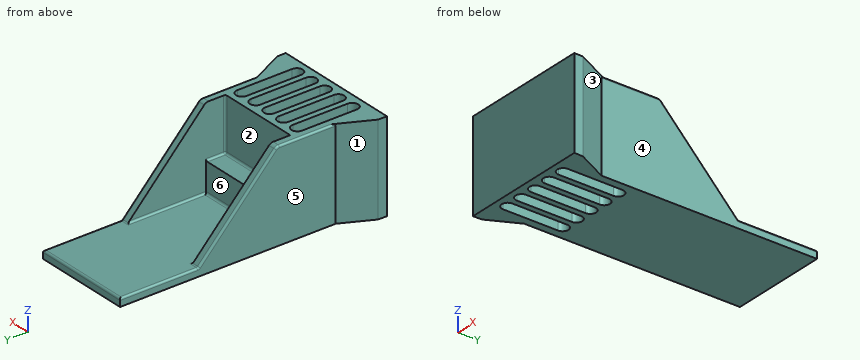
from build123d import *

# Parameters (mm, degrees)
SKETCH_1_W             = 50
SKETCH_1_H             = 46
EXTRUDE_1_DEPTH        = 40
EXTRUDE_2_DEPTH        = 10
SKETCH_8_W             = 42
SKETCH_8_H             = 10
EXTRUDE_5_DEPTH        = 15
SKETCH_3_W             = 50
SKETCH_3_H             = 4
EXTRUDE_3_DEPTH        = 80
SKETCH_4_W             = 70
SKETCH_4_H             = 46
SKETCH_5_W             = 50
SKETCH_5_H             = 46
EXTRUDE_4_DEPTH        = 4
FILLET_2_R             = 3
CHAMFER_1_SIZE2        = 2.113879869
CHAMFER_1_SIZE         = 5
CHAMFER_1_EDGE_2_SIZE2 = 5
CHAMFER_1_EDGE_2_SIZE  = 2.113879869
FILLET_4_R             = 1
CUT_EXTRUDE_1_DEPTH    = 47.0000001
FILLET_5_R             = 1


with BuildPart() as part:
    # 草图1 → 凸台-拉伸1 (new body)
    with BuildSketch(Plane(origin=(0, 0, 0), x_dir=(1, 0, 0), z_dir=(0, 1, 0))):
        with Locations((0, 2)):
            Rectangle(SKETCH_1_W, SKETCH_1_H)
    extrude(amount=EXTRUDE_1_DEPTH)

    # 草图2 → 凸台-拉伸2 (add)
    with BuildSketch(Plane(origin=(0, 40, 0), x_dir=(1, 0, 0), z_dir=(0, 1, 0))):
        Polygon((-25, 25), (-25, -21), (-21, -21), (-21, 21), (21, 21), (21, -21), (25, -21), (25, 25), align=None)
    extrude(amount=EXTRUDE_2_DEPTH)

    # 草图8 → 凸台-拉伸5 (add)
    with BuildSketch(Plane.XY.offset(-21)):
        with Locations((0, 45)):
            Rectangle(SKETCH_8_W, SKETCH_8_H)
    extrude(amount=EXTRUDE_5_DEPTH)

    # 草图3 → 凸台-拉伸3 (add)
    with BuildSketch(Plane(origin=(0, 50, 0), x_dir=(1, 0, 0), z_dir=(0, 1, 0))):
        with Locations((0, 23)):
            Rectangle(SKETCH_3_W, SKETCH_3_H)
    extrude(amount=EXTRUDE_3_DEPTH)

    # 草图4 → 放样2 section 0
    with BuildSketch(Plane.XZ):
        with Locations((0, -2)):
            Rectangle(SKETCH_4_W, SKETCH_4_H)
    # 草图5 → 放样2 section 1
    with BuildSketch(Plane(origin=(0, 20, 0), x_dir=(1, 0, 0), z_dir=(0, 1, 0))):
        with Locations((0, 2)):
            Rectangle(SKETCH_5_W, SKETCH_5_H)
    loft()

    # 草图6 → 凸台-拉伸4 (add)
    with BuildSketch(Plane.ZY.offset(25)):
        Polygon((-21, 90), (21, 50), (-21, 50), align=None)
    extrude_4 = extrude(amount=-EXTRUDE_4_DEPTH)

    # 镜向2: 凸台-拉伸4 across plane
    add(extrude_4.mirror(Plane(origin=(0, 0, 0), x_dir=(0, 0, 1), z_dir=(1, 0, 0))))

    # 圆角2
    fillet_2_edges = [part.edges().sort_by_distance(p)[0] for p in [
        (23, 50, 21),
        (-23, 50, 21),
    ]]
    fillet(fillet_2_edges, radius=FILLET_2_R)

    # 倒角1
    chamfer_1_edges = [part.edges().sort_by_distance(p)[0] for p in [
        (35, 0, -2),
    ]]
    chamfer(chamfer_1_edges, length=CHAMFER_1_SIZE, length2=CHAMFER_1_SIZE2)

    # 倒角1 edge 2
    chamfer_1_edge_2_edges = [part.edges().sort_by_distance(p)[0] for p in [
        (-35, 0, -2),
    ]]
    chamfer(chamfer_1_edge_2_edges, length=CHAMFER_1_EDGE_2_SIZE, length2=CHAMFER_1_EDGE_2_SIZE2)

    # 圆角4
    fillet_4_edges = [part.edges().sort_by_distance(p)[0] for p in [
        (21, 40, 7.5),
    ]]
    fillet(fillet_4_edges, radius=FILLET_4_R)

    # 草图7 → 切除-拉伸1 (cut, through all)
    with BuildSketch(Plane.XY.offset(21)):
        with BuildLine():
            Line((-21, 34), (-21, 6))
            ThreePointArc((-21, 6), (-18, 3), (-15, 6))
            Line((-15, 6), (-15, 34))
            ThreePointArc((-15, 34), (-18, 37), (-21, 34))
        make_face()
        with BuildLine():
            Line((-12, 34), (-12, 6))
            ThreePointArc((-12, 6), (-9, 3), (-6, 6))
            Line((-6, 6), (-6, 34))
            ThreePointArc((-6, 34), (-9, 37), (-12, 34))
        make_face()
        with BuildLine():
            Line((-3, 34), (-3, 6))
            ThreePointArc((-3, 6), (0, 3), (3, 6))
            Line((3, 6), (3, 34))
            ThreePointArc((3, 34), (0, 37), (-3, 34))
        make_face()
        with BuildLine():
            Line((6, 34), (6, 6))
            ThreePointArc((6, 6), (9, 3), (12, 6))
            Line((12, 6), (12, 34))
            ThreePointArc((12, 34), (9, 37), (6, 34))
        make_face()
        with BuildLine():
            Line((15, 34), (15, 6))
            ThreePointArc((15, 6), (18, 3), (21, 6))
            Line((21, 6), (21, 34))
            ThreePointArc((21, 34), (18, 37), (15, 34))
        make_face()
    extrude(amount=-CUT_EXTRUDE_1_DEPTH, mode=Mode.SUBTRACT)

    # 圆角5
    fillet_5_edges = [part.edges().sort_by_distance(p)[0] for p in [
        (-25, 34.357142857, 21),
        (25, 34.357142857, 21),
        (-25, 49.89604361, 20.75743509),
        (25, 49.89604361, 20.75743509),
        (-25, 70.443349754, -0.465517241),
        (25, 70.443349754, -0.465517241),
        (-0.5, 40, -6),
        (20.707106781, 40.292893219, -6),
        (21, 70, -21),
        (0, 50, -21),
        (-21, 70, -21),
        (-23, 90, -21),
        (-25, 110, -21),
        (0, 130, -21),
        (25, 110, -21),
        (23, 90, -21),
        (-21, 50, -13.5),
        (-21, 45, -6),
        (21, 45.5, -6),
    ]]
    fillet(fillet_5_edges, radius=FILLET_5_R)


solid = part.part
Here's how the part is built. I have some questions about the finished solid (model axes, mm). Face numbers are marked on the shaded views. A direction names the side the tool comes from. Give positions to 0.01 mm unless a question says otherwise; leave off trailing zeros. Loops run counter-clockwise (first coordinate to the right, second up) from the corner with the lowest first, then second, coordinate; pieces in that order, holes last. Notation, with made-up numbers: (-3.75, 83.25) -> (43.25, 83.25) arc R25 ccw to (43.25, 109.25) -> close; hole circle Ø2 at (32.25, 22). An arc over 180 degrees is marked (long way). Answer as a JSON object with one key per item and string values. Group by question number.
Item 1: Will these pins go through, and if not, where does the flat tip stop? pin 1 (8 mm diameter, centred on x = 0.5, z = 9.5, fed in from +Y); pin 2 (8.5 mm diameter, centred on y = 26.5, z = -11.5, fed in from -X); pin 3 (10 mm diameter, centred on x = 5, y = 47, fed in from +Z); pin 4 (16.5 mm diameter, centred on x = 2, z = -16, fed in from +Y).
Item 2: Imagine slicing it at A-A on y = 24. Write out the boundary of the cut face in (x, z).
Item 3: Imagine slicing it at D-D on z = -2. Give the number of separate pieces and of enclosed holes in the cut face, then the cut area to 3 significant figures.
Item 4: Thinking about a two-plate mould opening in X: for the marked faces 1, 2 and 3, which applies, pulls with the +X half, pulls with the -X half, needs draft (parallel to the pull), parting line crosses it, or undercut?
Item 5: On a 3-axis mill with a long thin cutter (end or side, diameter ignored), from which of +Z, -Z, +X, -X, +Y, -Y can I reach the whole of each face in a straight line? I mean the marked faces 4, 5 and 6. Say none if no direction works.
Item 6: I need wall thicknesses on L1, parallel to X at y = 64, z = -15; L2, parallel to X at y = 31, z = -22; L3, parallel to Z at x = -11, y = 47. Which ranges of each line are inside material? Lowest first, please.
Item 7: Imagine slicing it at B-B on x = 9. Write out the boundary of the cut face in (y, z), then the cut area to 3 significant figures.
Item 8: Imagine slicing it at C-C on y = 117.5. Write out the boundary of the cut face in (x, z).
Answer list:
{
 "1": {"pin 1": "stops at y = 40", "pin 2": "stops at x = -25", "pin 3": "stops at z = -6", "pin 4": "stops at y = 130"},
 "2": {"outline": "(-25, -25) -> (-21, -25) -> (-21, 21) -> (-24, 21) arc R1 ccw to (-25, 20) -> close; (-15, -25) -> (-12, -25) -> (-12, 21) -> (-15, 21) -> close; (-6, -25) -> (-3, -25) -> (-3, 21) -> (-6, 21) -> close; (3, -25) -> (6, -25) -> (6, 21) -> (3, 21) -> close; (12, -25) -> (15, -25) -> (15, 21) -> (12, 21) -> close; (21, -25) -> (25, -25) -> (25, 20) arc R1 ccw to (24, 21) -> (21, 21) -> close"},
 "3": {"separate pieces": "1", "enclosed holes": "5", "area": "1,460 mm2"},
 "4": {"face 1": "pulls with the -X half", "face 2": "undercut", "face 3": "pulls with the +X half"},
 "5": {"face 4": "+Z, -Z, +X, +Y", "face 5": "+Z, -Z, -X, +Y", "face 6": "+Z, +Y"},
 "6": {"L1": "x = -25 to -21, 21 to 25", "L2": "x = -25 to -21, -15 to -12, -6 to -3, 3 to 6, 12 to 15, 21 to 25", "L3": "z = -25 to -6"},
 "7": {"outline": "(0, -25) -> (3, -25) -> (3, 21) -> (0, 21) -> close; (37, -25) -> (130, -25) -> (130, -22) arc R1 ccw to (129, -21) -> (51, -21) arc R1 cw to (50, -20) -> (50, -6) -> (41, -6) arc R1 cw to (40, -5) -> (40, 21) -> (37, 21) -> close", "area": "786 mm2"},
 "8": {"outline": "(-25, -25) -> (25, -25) -> (25, -22) arc R1 ccw to (24, -21) -> (-24, -21) arc R1 ccw to (-25, -22) -> close"}
}
